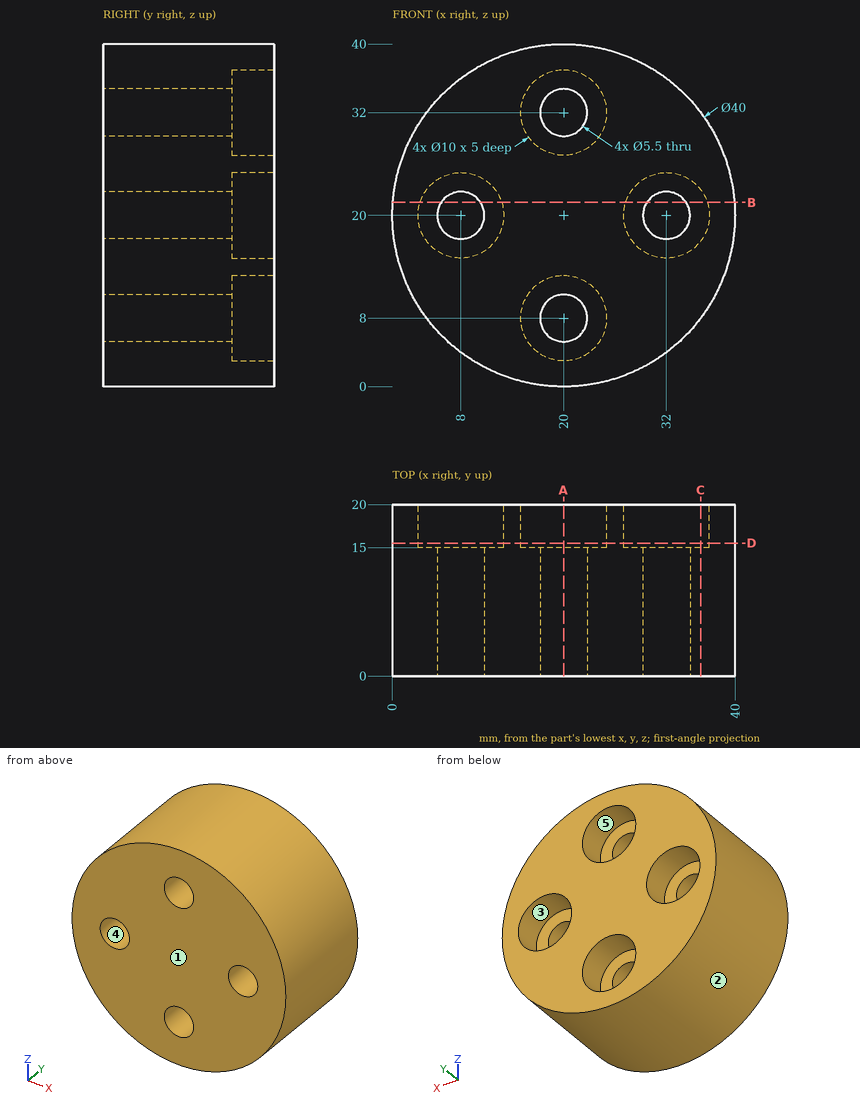
Design review of the part shown in the three views and the two pictorial views. Dimensions are in mm from the part's minimum x, y and z. A direction names the side the tool comes from. Round coordinates to 2 decimals unless told otherwise and drop trailing zeros. Loops run counter-clockwise (first coordinate to the right, second up) from the corner with the lowest first, then second, coordinate; pieces in that order, holes last. Notation, with made-up numbers: M 26,60.25 L 78,60.25 A23 cw 78,73.25 Z; hole C 40,70 d8. An arc over 180 degrees is marked long. Answer as a JSON object with one key per item and string values.
Item 1: Tool access review of the marked faces 4 and 5: name each direction out of +Z, -Z, +X, -X, +Y, -Y from which nothing blocks a thin tool from reaching the whole face with its end or side.
Check sheet entries:
{"face 4": "+Y, -Y", "face 5": "+Y"}
Item 2: For line 1 along X through (y, z) = (8.5, 20); line 2 along X through (y, z) = (10.5, 18.5); line 3 along Z through (x, y) = (21, 12.5), list the stretches that pass through material, from the lowest coordinate up.
Check sheet entries:
{"line 1": "0 to 5.25, 10.75 to 29.25, 34.75 to 40", "line 2": "0.06 to 5.7, 10.3 to 29.7, 34.3 to 39.94", "line 3": "0.03 to 5.44, 10.56 to 29.44, 34.56 to 39.97"}
Item 3: We need section A-A, the plane x = 20. State the section outline as (y, z) points, and give its area (3 significant figures).
Check sheet entries:
{"outline": "M 0,0 L 20,0 L 20,3 L 15,3 L 15,5.25 L 0,5.25 Z; M 0,10.75 L 15,10.75 L 15,13 L 20,13 L 20,27 L 15,27 L 15,29.25 L 0,29.25 Z; M 0,34.75 L 15,34.75 L 15,37 L 20,37 L 20,40 L 0,40 Z", "area": "535 mm2"}
Item 4: We need section D-D, the plane y = 15.5. State the section outline as (x, z) points.
Check sheet entries:
{"outline": "C 20,20 d40; hole C 8,20 d10; hole C 20,8 d10; hole C 20,32 d10; hole C 32,20 d10"}
Item 5: The part is to be moulded in two halves that separate along Z. For the marked faces 1, 2 and 3, say which applies: +Z half, -Z half, draft (parallel to the pull), parting line (faces both ways), or undercut.
Check sheet entries:
{"face 1": "draft", "face 2": "parting line", "face 3": "undercut"}
Item 6: We need section B-B, the plane z = 21.5. State the section outline as (x, y) points, and give its area (3 significant figures).
Check sheet entries:
{"outline": "M 0.06,0 L 5.7,0 L 5.7,15 L 3.23,15 L 3.23,20 L 0.06,20 Z; M 10.3,0 L 29.7,0 L 29.7,15 L 27.23,15 L 27.23,20 L 12.77,20 L 12.77,15 L 10.3,15 Z; M 34.3,0 L 39.94,0 L 39.94,20 L 36.77,20 L 36.77,15 L 34.3,15 Z", "area": "564 mm2"}
Item 7: Clearance check with flat-ended pins moving along their axes: P1, Ø6.5, axis at x = 20, z = 32, coming from the +Y side; P2, Ø12, axis at x = 27.5, y = 12, coming from the -Z side; P3, Ø4, axis at x = 4.5, y = 4.5, coming from the -Z side; P4, Ø4.5, axis at x = 20, z = 8, coming from the -Y side. State where each tip first meets the part, or that it passes through.
Check sheet entries:
{"P1": "y = 15", "P2": "z = 0.06", "P3": "z = 5.24", "P4": "through"}
Item 8: We need section C-C, the plane x = 36. State the section outline as (y, z) points.
Check sheet entries:
{"outline": "M 0,8 L 20,8 L 20,17 L 15,17 L 15,23 L 20,23 L 20,32 L 0,32 Z"}
